```python
from build123d import *

# Parameters (mm, degrees)
F0_R     = 63.5
F1_DEPTH = 12.7
F4_R     = 50.8
F5_DEPTH = 25.4
F6_R     = 38.1
F7_DEPTH = 38.1
F8_R     = 25.4
F9_DEPTH = 50.8
F10_R    = 5.08
F11_R    = 5.08
F12_R    = 5.08


# Not quite as in the source:
# - the program builds the solid bodies; features that only make, move or delete a surface that nothing else refers to are left out


with BuildPart() as f1:
    # F0 (on Top) → F1 (new body)
    with BuildSketch(Plane.XY):
        Circle(F0_R)
    extrude(amount=F1_DEPTH)

    # F4 (on Top) → F5 (join)
    with BuildSketch(Plane.XY):
        Circle(F4_R)
    extrude(amount=F5_DEPTH)

    # F6 (on Top) → F7 (join)
    with BuildSketch(Plane.XY):
        Circle(F6_R)
    extrude(amount=F7_DEPTH)

    # F8 (on Top) → F9 (join)
    with BuildSketch(Plane.XY):
        Circle(F8_R)
    extrude(amount=F9_DEPTH)

    # F10
    f10_edges = [f1.edges().sort_by_distance(p)[0] for p in [
        (-25.4, 0, 50.8),
    ]]
    fillet(f10_edges, radius=F10_R)

    # F11
    f11_edges = [f1.edges().sort_by_distance(p)[0] for p in [
        (-38.1, 0, 38.1),
    ]]
    fillet(f11_edges, radius=F11_R)

    # F12
    f12_edges = [f1.edges().sort_by_distance(p)[0] for p in [
        (-50.8, 0, 25.4),
    ]]
    fillet(f12_edges, radius=F12_R)


solid = f1.part
```
For this review, take the finished solid that the model builds, in its own axes (mm). A direction names the side the tool comes from. Round coordinates to 2 decimals unless told otherwise and drop trailing zeros. Write each loop counter-clockwise with the first axis right and the second up, starting at its lowest first coordinate (ties: lowest second). Pieces come first, ordered by that corner, then holes. Notation, with made-up numbers: (-14.75, -25) - (-5.75, -25) arc R24 ccw to (-5.75, -8) - close; hole circle Ø1 at (20, 46). An arc over 180 degrees is marked (long way). Answer as CSV lines item,"result". Start each with the question number.
(1) Add section A-A, the plane x = 0. State the section outline as (y, z) points, plus the area to 3 significant figures.
(2) For line 1 (Z direction, x = 27, y = -51.5); line 2 (Z direction, x = 29, y = -29.5); line 3 (X direction, y = 9, z = 36), list the stretches that pass through material, from the lowest coordinate up.
(3) Machinability: for faces 1 (the flat face through (-29, 43, 12.7)), 2 (the flat face through (-1, 1, 0)), which of the approach directions +Z, -Z, +X, -X, +Y, -Y give a long, thin tool a straight path to every point of the face, cutting with its end or side? Answer none if there is none.
(4) Add section C-C, the plane z = 4. State the section outline as (x, y) points.
(5) For pin 1 (1 mm diameter, centred on y = 13.5, z = 41, fed in from -X); pin 2 (10 mm diameter, centred on y = 20.5, z = 40, fed in from +X); pin 3 (8 mm diameter, centred on x = 25.5, z = 19.5, fed in from -Y), all flat-tipped, find the tip position at first contact; note any pin that passes through.
From the geometry:
1,outline,"(-63.5, 0) - (63.5, 0) - (63.5, 12.7) - (50.8, 12.7) - (50.8, 20.32) arc R5.08 ccw to (45.72, 25.4) - (38.1, 25.4) - (38.1, 33.02) arc R5.08 ccw to (33.02, 38.1) - (25.4, 38.1) - (25.4, 45.72) arc R5.08 ccw to (20.32, 50.8) - (-20.32, 50.8) arc R5.08 ccw to (-25.4, 45.72) - (-25.4, 38.1) - (-33.02, 38.1) arc R5.08 ccw to (-38.1, 33.02) - (-38.1, 25.4) - (-45.72, 25.4) arc R5.08 ccw to (-50.8, 20.32) - (-50.8, 12.7) - (-63.5, 12.7) - close"
1,area,"4,480 mm²"
2,line 1,"z = 0 to 12.7"
2,line 2,"z = 0 to 25.4"
2,line 3,"x = -36.03 to 36.03"
3,face 1,"+Z"
3,face 2,"-Z, +X, -X, +Y, -Y"
4,outline,"circle Ø127 at (0, 0)"
5,pin 1,"stops at x = -21.82"
5,pin 2,"stops at x = 32.76"
5,pin 3,"stops at y = -46.03"
